Build history of the part. All positions in model axes, mm. A direction names the side the tool comes from. Round coordinates to 2 decimals unless told otherwise and drop trailing zeros. Order: outer loops, then holes, each group sorted by start corner. A loop starts at its lowest first (then second) coordinate and runs counter-clockwise, first axis right, second up. Notation, with made-up numbers: M -39.5,-36 L 8.5,-36 A16 cw 8.5,-27 Z; hole C -19.75,26.25 d2. An arc over 180 degrees is marked long. One line per item, written item: value. Start each with the question number.
Item 1: Pin check, flat tips, straight feed: pin 1 (2.5 mm diameter, centred on x = -1.5, y = 1, fed in from +Z); pin 2 (3 mm diameter, centred on y = -2, z = -3.5, fed in from +X); pin 3 (4 mm diameter, centred on x = 2.5, z = -60, fed in from +Y); pin 4 (4 mm diameter, centred on x = -2.5, z = -63, fed in from +Y). Stop position of each tip, or through.
Item 2: Two-plate mould, pull along X, no slides. Class faces 1 (the flat face through (-1, 2, -63.1)), 2 (the flat face through (0, 0, -10)), 3 (the cylindrical face through (-5.052, -1.122, -24.206)): +X half, -X half, draft (parallel to the pull), parting line (faces both ways), or undercut.
Item 3: Tool access for faces 4 (the cylindrical face through (-3.38, 0.49, -5.55)), 5 (the flat face through (-2, 0, -49.1)), 6 (the flat face through (-1.625, 0, -6)), 7 (the flat face through (-3, 0, 0)), 8 (the cylindrical face through (-3.905, -0.867, -67.044)): list every direction of +Z, -Z, +X, -X, +Y, -Y with a clear straight run to the whole face (end or side of a thin tool).
Item 4: Band-saw the part on B-B, the plane y = 0.75. Write the cut outline in (x, z) (3 decimals), then the cut area to 3 significant figures.
Item 5: Band-saw the part on A-A, the plane z = -4. Write the cut outline in (x, y) (3 decimals).
Item 6: Probe L1, parallel to Z at x = -3, y = 0 (3 decimals); L2, parallel to Z at x = 1.5, y = -1; L3, parallel to Z at x = -4.3, y = 0 (3 decimals). List the from-to ranges inside material, lowest first.
Item 7: Band-saw the part on D-D, the plane z = -35.5. Write the cut outline in (x, y) (3 decimals).
Item 8: Band-saw the part on C-C, the plane x = -2.5. Give the number of separate pieces and of enclosed holes in the cut face, then the cut area to 3 significant figures.
```python
from build123d import *

# Parameters (mm, degrees)
SKETCH1_W          = 14
SKETCH1_H          = 1.75
SKETCH4_W          = 3.25
SKETCH4_H          = 11
CUT_EXTRUDE1_DEPTH = 10
SKETCH5_R          = 1.625
CUT_EXTRUDE2_DEPTH = 12


with BuildPart() as part:
    # Sketch1 → Revolve1 (revolve)
    with BuildSketch(Plane(origin=(0, 0, 0), x_dir=(0, 0, -1), z_dir=(1, 0, 0))):
        Polygon((0, 5.175), (0, 0), (49.1, 0), (49.1, 1.75), (49.1, 5.175), align=None)
        with Locations((56.1, 0.875)):
            Rectangle(SKETCH1_W, SKETCH1_H)
        Polygon((63.1, 1.75), (63.1, 0), (71.1, 0), (71.1, 4), (63.1, 4), align=None)
    revolve(axis=Axis((0, 0, -49.1), (0, 0, -1)))

    # Sketch4 → Cut-Extrude1 (cut)
    with BuildSketch(Plane.XY):
        Rectangle(SKETCH4_W, SKETCH4_H)
    extrude(amount=-CUT_EXTRUDE1_DEPTH, mode=Mode.SUBTRACT)

    # Sketch5 → Cut-Extrude2 (cut)
    with BuildSketch(Plane(origin=(5.175, 0, 0), x_dir=(0, 0, -1), z_dir=(1, 0, 0))):
        with Locations((4, 0)):
            Circle(SKETCH5_R)
    extrude(amount=-CUT_EXTRUDE2_DEPTH, mode=Mode.SUBTRACT)


solid = part.part
```
Output:
1. pin 1: stops at z = 0
1. pin 2: stops at x = 5.11
1. pin 3: stops at y = 1.68
1. pin 4: stops at y = 3.97
2. face 1: draft
2. face 2: undercut
2. face 3: parting line
3. face 4: +X, -X
3. face 5: none
3. face 6: +Z, +Y, -Y
3. face 7: +Z, +X, -X, +Y, -Y
3. face 8: -Z
4. outline: M -5.12,-49.1 L -1.581,-49.1 L -1.581,-63.1 L -3.929,-63.1 L -3.929,-71.1 L 3.929,-71.1 L 3.929,-63.1 L 1.581,-63.1 L 1.581,-49.1 L 5.12,-49.1 L 5.12,-5.442 L 1.625,-5.442 L 1.625,-10 L -1.625,-10 L -1.625,-5.442 L -5.12,-5.442 Z; M -5.12,-2.558 L -1.625,-2.558 L -1.625,0 L -5.12,0 Z; M 1.625,-2.558 L 5.12,-2.558 L 5.12,0 L 1.625,0 Z
4. area: 557 mm²
5. outline: M -4.913,-1.625 A5.175 ccw -1.625,-4.913 L -1.625,-1.625 Z; M -4.913,1.625 L -1.625,1.625 L -1.625,4.913 A5.175 ccw Z; M 1.625,-4.913 A5.175 ccw 4.913,-1.625 L 1.625,-1.625 Z; M 1.625,1.625 L 4.913,1.625 A5.175 ccw 1.625,4.913 Z
6. L1: z = -71.1 to -63.1, -49.1 to -5.625, -2.375 to 0
6. L2: z = -71.1 to -63.1, -49.1 to -10
6. L3: z = -49.1 to -5.625, -2.375 to 0
7. outline: C 0,0 d10.35
8. separate pieces: 2
8. enclosed holes: 1
8. area: 487 mm²
